Here's how the part is built. I have some questions about the finished solid (model axes, mm). Face numbers are marked on the shaded views. A direction names the side the tool comes from. Round coordinates to 2 decimals unless told otherwise and drop trailing zeros. Loops run counter-clockwise (first coordinate to the right, second up) from the corner with the lowest first, then second, coordinate; pieces in that order, holes last. Notation, with made-up numbers: M 34.5,86.25 L 62.5,86.25 A13 ccw 62.5,96.25 Z; hole C -5.5,33.25 d3. An arc over 180 degrees is marked long. Use a Markdown table: item, result.
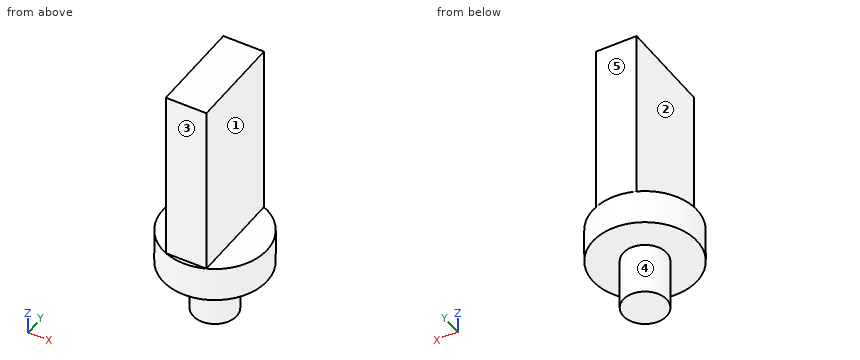
from build123d import *

# Parameters (mm, degrees)
F0_R     = 1.25
F1_DEPTH = 3
F2_R     = 3
F3_DEPTH = 2
F4_W     = 2.331915
F4_H     = 5.528303
F5_DEPTH = 10


with BuildPart() as f1:
    # F0 (on Top) → F1 (new body)
    with BuildSketch(Plane.XY):
        Circle(F0_R)
    extrude(amount=F1_DEPTH)

    # F2 (on face) → F3 (join)
    with BuildSketch(Plane.XY.offset(3)):
        Circle(F2_R)
    extrude(amount=F3_DEPTH)

    # F4 (on face) → F5 (join)
    with BuildSketch(Plane.XY.offset(5)):
        with Locations((-0.003007, -0.001268)):
            Rectangle(F4_W, F4_H)
    extrude(amount=F5_DEPTH)


solid = f1.part
1. Imagine slicing it at A-A, the plane x = 0. Write out the boundary of the cut face in (y, z).
Answer sheet:
| item | result |
|---|---|
| outline | M -3,3 L -1.25,3 L -1.25,0 L 1.25,0 L 1.25,3 L 3,3 L 3,5 L 2.76,5 L 2.76,15 L -2.77,15 L -2.77,5 L -3,5 Z |
2. For pin 1 Ø1.7 at (y, z) = (-1, 8.5) entering from -X; pin 2 Ø2.5 at (x, z) = (0.5, 7.5) entering from -Y; pin 3 Ø1 at (x, z) = (2, 6.5) entering from +Y; pin 4 Ø3 at (y, z) = (-0.5, 11.5) entering from +X, each with a flat end and sliding along its axis, tell me the tip position at first contact or that it passes through.
Answer sheet:
| item | result |
|---|---|
| pin 1 | x = -1.17 |
| pin 2 | y = -2.77 |
| pin 3 | through |
| pin 4 | x = 1.16 |
3. Which directions (+Z, -Z, +X, -X, +Y, -Y) give clear straight access to the entire face, cutting with the end or side of a thin tool? Please do the marked faces 1, 2, 3, 4 and 5.
Answer sheet:
| item | result |
|---|---|
| face 1 | +Z, +X, +Y, -Y |
| face 2 | +Z, -X, +Y, -Y |
| face 3 | +Z, +X, -X, -Y |
| face 4 | -Z |
| face 5 | +Z, +X, -X, +Y |
4. Imagine slicing it at D-D, the plane y = -1.95. Write out the boundary of the cut face in (x, z).
Answer sheet:
| item | result |
|---|---|
| outline | M -2.28,3 L 2.28,3 L 2.28,5 L 1.16,5 L 1.16,15 L -1.17,15 L -1.17,5 L -2.28,5 Z |
5. Imagine slicing it at B-B, the plane y = 0. Write out the boundary of the cut face in (x, z).
Answer sheet:
| item | result |
|---|---|
| outline | M -3,3 L -1.25,3 L -1.25,0 L 1.25,0 L 1.25,3 L 3,3 L 3,5 L 1.16,5 L 1.16,15 L -1.17,15 L -1.17,5 L -3,5 Z |
6. Imagine slicing it at C-C, the plane z = 2.5. Write out the boundary of the cut face in (x, y), then the cut area to 3 significant figures.
Answer sheet:
| item | result |
|---|---|
| outline | C 0,0 d2.5 |
| area | 4.91 mm2 |
7. I need wall thicknesses on probe 1 along Y at (x, z) = (-0.2, 8.25); probe 2 along X at (y, z) = (-2.65, 10.5); probe 3 along Z at (x, y) = (1.35, -1). Which ranges of each line are inside material? Lowest first, please. Write a range as from..to.
Answer sheet:
| item | result |
|---|---|
| probe 1 | -2.77..2.76 |
| probe 2 | -1.17..1.16 |
| probe 3 | 3..5 |
